Source: CAD feature listing. Evaluate the final solid. Frame: model axes, mm. Face numbers are marked on the shaded views. Give positions to 0.01 mm unless a question says otherwise; leave off trailing zeros. Loops run counter-clockwise (first coordinate to the right, second up) from the corner with the lowest first, then second, coordinate; pieces in that order, holes last. Notation, with made-up numbers: (26, -16) - (47, -16) arc R34 cw to (47, 22) - close; hole circle Ø3 at (10, 26.25). An arc over 180 degrees is marked (long way). Write each question's results on one line, items separated by ' | '. Start each with the question number.
(1) Cut plane A-A on y = 3.5. Return the cut outline in (x, z).
(2) Material intervals for line 1 along Y through (x, z) = (-16.5, 19.25); line 2 along Y through (x, z) = (-35.5, 13); line 3 along X through (y, z) = (-3.5, 6), sorted ascending. Write a range as [from, to].
(3) Contact query for flat-ended pins moving along their axis: pin 1 (4 mm diameter, centred on x = -12, z = 16.5, fed in from +Y); pin 2 (5 mm diameter, centred on y = 9.79, z = 12.5, fed in from -X); pin 3 (4 mm diameter, centred on y = 4, z = 3, fed in from -X). Output: stop coordinate, or through.
(4) Pull-direction query (Y, two-part tool) for the marked faces 1, 2, 3 and 4; classes: pulls with the +Y half, pulls with the -Y half, needs draft (parallel to the pull), parting line crosses it, or undercut.
from build123d import *

# Parameters (mm, degrees)
F1_DEPTH    = 25
F2_T1_DEPTH = 30.6274350033
F2_T3_DEPTH = 31.8341602247
F3_T        = -2.5
F4_DEPTH    = 25
F6_DEPTH    = 3
F7_SIZE     = 1.2


# Not quite as in the source:
# - a fillet or chamfer that OpenCascade refuses, or shapes differently, is made with other operations: its cross-section is extruded or revolved along the edge and cut away or added


with BuildPart() as f1:
    # F0 (on Top) → F1 (new body)
    with BuildSketch(Plane.XY):
        with BuildLine():
            Line((0, -23.9775525033), (0, 0))
            Line((0, 0), (0, 26.0224474967))
            add(Edge.make_bspline(
                [(0, 26.0224474967), (-18.2413181838, 20.2646104982), (-36.4872975651, 14.5034889639), (-42.1967271812, 16.6896569806)],
                knots=[0, 0, 0, 0, 0.7457520739, 0.7457520739, 0.7457520739, 0.7457520739], degree=3))
            ThreePointArc((-42.1967271812, 16.6896569806), (-46.7941768856, 7.5931695596), (-56.9807893445, 7.2532375123))
            Line((-56.9807893445, 7.2532375123), (0, -23.9775525033))
        make_face()
        with BuildLine():
            ThreePointArc((-56.9807893445, 7.2532375123), (-46.7941768856, 7.5931695596), (-42.1967271812, 16.6896569806))
            Line((-42.1967271812, 16.6896569806), (-43.6933846934, 16.589575558))
            ThreePointArc((-43.6933846934, 16.589575558), (-54.7874105132, 7.9340356852), (-58.7207947374, 21.4441899376))
            Line((-58.7207947374, 21.4441899376), (-59.8760331153, 22.4009680155))
            ThreePointArc((-59.8760331153, 22.4009680155), (-61.9966403153, 14.1450934668), (-56.9807893445, 7.2532375123))
        make_face()
    extrude(amount=F1_DEPTH)

    # F2: fillet of radius 1.2 on 3 edges, made by hand

    # F2_s2 → F2_t1 (cut)
    with BuildSketch(Plane.XY.offset(-2.8137175017)):
        with BuildLine():
            ThreePointArc((-59.3412383143, 20.5926836221), (-59.1675384199, 21.4239873058), (-59.5875985888, 22.1620841304))
            Line((-59.5875985888, 22.1620841304), (-58.7207947374, 21.4441899376))
            ThreePointArc((-58.7207947374, 21.4441899376), (-59.0442222025, 21.0280589954), (-59.3412383143, 20.5926836221))
        make_face()
        with BuildLine():
            ThreePointArc((-42.5704056438, 16.6646691181), (-43.3428946364, 16.3118260592), (-43.6883739189, 15.5360158161))
            ThreePointArc((-43.6883739189, 15.5360158161), (-43.6745400624, 16.0628733972), (-43.6933846934, 16.589575558))
            Line((-43.6933846934, 16.589575558), (-42.5704056438, 16.6646691181))
        make_face()
    extrude(amount=F2_T1_DEPTH, mode=Mode.SUBTRACT)

    # F2_s4 → F2_t3 (cut)
    with BuildSketch(Plane.XY.offset(-3.4170801123)):
        with BuildLine():
            ThreePointArc((-58.8885337226, 21.5831127668), (-59.8476100394, 21.8431932263), (-60.6738896743, 21.2911685965))
            ThreePointArc((-60.6738896743, 21.2911685965), (-60.2939449544, 21.8597159591), (-59.8760331153, 22.4009680155))
            Line((-59.8760331153, 22.4009680155), (-58.8885337226, 21.5831127668))
        make_face()
    extrude(amount=F2_T3_DEPTH, mode=Mode.SUBTRACT)

    # F3
    f3_openings = [f1.faces().sort_by_distance(p)[0] for p in [
        (-19.977186, 3.669983, 25),
    ]]
    offset(amount=F3_T, openings=f3_openings)

    # F4 (cut): a face of the model
    f4_faces = [f1.faces().sort_by_distance(p)[0] for p in [
        (-18.9574034875, 3.5679781743, 2.5),
    ]]
    extrude(f4_faces, amount=-F4_DEPTH, mode=Mode.SUBTRACT)

    # F5 (on face) → F6 (cut)
    with BuildSketch(Plane.YZ):
        with BuildLine():
            ThreePointArc((12.9166145043, 10), (13.5683701333, 11.1752351146), (13.7941155051, 12.5))
            ThreePointArc((13.7941155051, 12.5), (13.5683701333, 13.8247648854), (12.9166145043, 15))
            ThreePointArc((12.9166145043, 15), (5.7941155051, 12.5), (12.9166145043, 10))
        make_face()
        with BuildLine():
            ThreePointArc((20.5641841143, 12.5), (19.8319510673, 14.267766953), (18.0641841143, 15))
            ThreePointArc((18.0641841143, 15), (15.5641841143, 12.5), (18.0641841143, 10))
            ThreePointArc((18.0641841143, 10), (19.8319510673, 10.732233047), (20.5641841143, 12.5))
        make_face()
        with BuildLine():
            ThreePointArc((12.9166145043, 15), (13.5683701333, 13.8247648854), (13.7941155051, 12.5))
            ThreePointArc((13.7941155051, 12.5), (13.5683701333, 11.1752351146), (12.9166145043, 10))
            Line((12.9166145043, 10), (18.0641841143, 10))
            ThreePointArc((18.0641841143, 10), (15.5641841143, 12.5), (18.0641841143, 15))
            Line((18.0641841143, 15), (12.9166145043, 15))
        make_face()
    extrude(amount=-F6_DEPTH, mode=Mode.SUBTRACT)

    # F7
    f7_edges = [f1.edges().sort_by_distance(p)[0] for p in [
        (-2.5, 15.490399, 10),
        (-2.5, 15.490399, 15),
        (-2.5, 20.564184, 12.5),
    ]]
    chamfer(f7_edges, length=F7_SIZE)


solid = f1.part
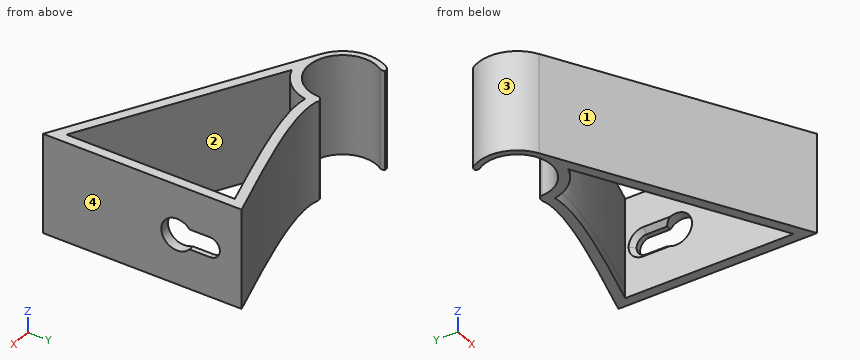
Ans:
1) outline: (-50.13, 0) - (-44.93, 0) - (-44.93, 25) - (-50.13, 25) - close; (-2.5, 0) - (0, 0) - (0, 25) - (-2.5, 25) - close
2) line 1: [-14.93, -12.08], [18.33, 20.93] | line 2: [-4.52, -1.67], [13.93, 16.45] | line 3: [-37.36, -32.16], [-2.5, 0]
3) pin 1: y = 22.89 | pin 2: x = -61.45 | pin 3: x = -54.69
4) face 1: pulls with the -Y half | face 2: undercut | face 3: parting line crosses it | face 4: needs draft
